Drawing for the job (mm, zero at the part's lowest x, y, z). Coordinates: 2 decimals unless noted, no trailing zeros. Order: outer loops, then holes, each group sorted by start corner. A loop starts at its lowest first (then second) coordinate and runs counter-clockwise, first axis right, second up.
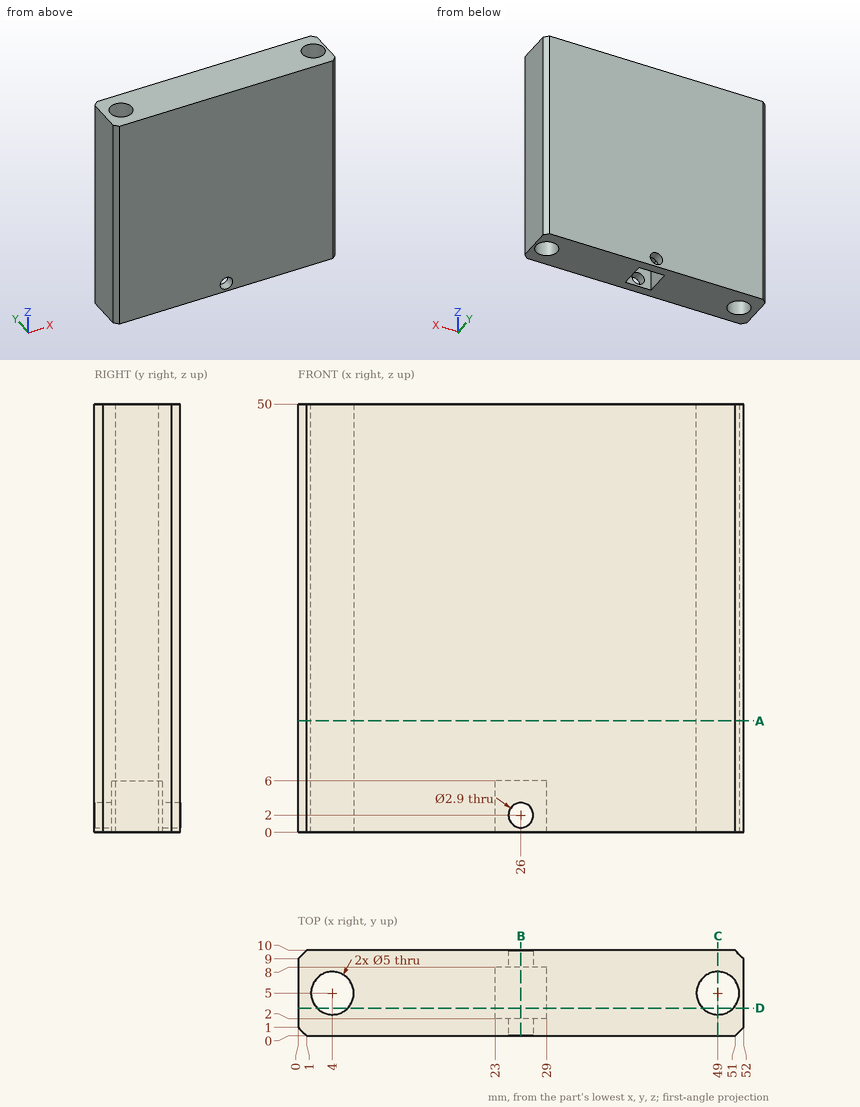
(1) Slice it at C-C, the plane x = 49. Give the cut face in (y, z), then the cut area to 3 significant figures.
(2) Slice it at B-B, the plane x = 26. Give the cut face in (y, z), then the cut area to 3 significant figures.
(3) Slice it at D-D, the plane y = 3.25. Give the cut face in (x, z).
(4) Drop a flat-ended pin along its axis: pin 1 (3 mm diameter, centred on x = 26, y = 4.5, fed in from -Z). Give the stop position or say it passes through.
(5) Slice it at A-A, the plane z = 13. Give the cut face in (x, y).
(6) Probe line 1 (X direction, y = 1.25, z = 2); line 2 (X direction, y = 6.25, z = 9); line 3 (Y direction, x = 5.5, z = 4). List the from-to ranges inside material, lowest first.
Here are the results:
1. outline: (0, 0) - (2.5, 0) - (2.5, 50) - (0, 50) - close; (7.5, 0) - (10, 0) - (10, 50) - (7.5, 50) - close
1. area: 250 mm2
2. outline: (0, 0) - (2, 0) - (2, 0.55) - (0, 0.55) - close; (0, 3.45) - (2, 3.45) - (2, 6) - (8, 6) - (8, 3.45) - (10, 3.45) - (10, 50) - (0, 50) - close; (8, 0) - (10, 0) - (10, 0.55) - (8, 0.55) - close
2. area: 452 mm2
3. outline: (0, 0) - (2.21, 0) - (2.21, 50) - (0, 50) - close; (5.79, 0) - (23, 0) - (23, 6) - (29, 6) - (29, 0) - (47.21, 0) - (47.21, 50) - (5.79, 50) - close; (50.79, 0) - (52, 0) - (52, 50) - (50.79, 50) - close
4. pin 1: stops at z = 6
5. outline: (0, 1) - (1, 0) - (51, 0) - (52, 1) - (52, 9) - (51, 10) - (1, 10) - (0, 9) - close; hole circle Ø5 at (4, 5); hole circle Ø5 at (49, 5)
6. line 1: x = 0 to 24.55, 27.45 to 52
6. line 2: x = 0 to 1.83, 6.17 to 46.83, 51.17 to 52
6. line 3: y = 0 to 3, 7 to 10
